For this review, take the finished solid that the model builds, in its own axes (mm). Face numbers are marked on the shaded views. A direction names the side the tool comes from. Coordinates: 2 decimals unless noted, no trailing zeros. Write each loop counter-clockwise with the first axis right and the second up, starting at its lowest first coordinate (ties: lowest second). Pieces come first, ordered by that corner, then holes. Notation, with made-up numbers: M 69,1.5 L 118,1.5 A21 cw 118,25.5 Z; hole C -15.5,61 d4. An arc over 180 degrees is marked long. One line per question, with ' | ' between items.
from build123d import *

# Parameters (mm, degrees)
ESQUISSE2_R             = 65
ESQUISSE2_R_2           = 44
BOSS_EXTRU_1_START      = -47
ESQUISSE3_R             = 112.5
ESQUISSE3_R_2           = 44
BOSS_EXTRU_1_DEPTH      = 47
ENL_V_START             = -10
ESQUISSE4_R             = 112.5
ESQUISSE4_R_2           = 65
ENL_V_MAT_EXTRU_1_DEPTH = 10
ESQUISSE5_R             = 112.5
ESQUISSE5_R_2           = 44
BOSS_EXTRU_2_DEPTH      = 37


with BuildPart() as part:
    # Balayage-Mince1: sweep along a path in Esquisse1
    with BuildLine(Plane(origin=(0, 0, 0), x_dir=(0, 0, -1), z_dir=(1, 0, 0))) as balayage_mince1_path:
        Line((0, 0), (-47, 0))
        ThreePointArc((-47, 0), (-133.103772282, 17.127105185), (-206.099025767, 65.900974233))
        Line((-206.099025767, 65.900974233), (-232.261976671, 92.063925137))
    # Esquisse2 → Balayage-Mince1 (sweep)
    with BuildSketch(Plane.XY):
        Circle(ESQUISSE2_R)
        Circle(ESQUISSE2_R_2, mode=Mode.SUBTRACT)
    sweep(path=balayage_mince1_path.line)

    # Esquisse3 → Boss.-Extru.1 (add)
    with BuildSketch(Plane(origin=(0, 0, 0), x_dir=(-1, 0, 0), z_dir=(0, 0, -1)).offset(BOSS_EXTRU_1_START)):
        Circle(ESQUISSE3_R)
        with Locations(Location((0, 0, 0), (0, 0, 180))):
            Circle(ESQUISSE3_R_2, mode=Mode.SUBTRACT)
    extrude(amount=BOSS_EXTRU_1_DEPTH)

    # Esquisse4 → Enlèv. mat.-Extru.1 (cut)
    with BuildSketch(Plane(origin=(0, 0, 0), x_dir=(-1, 0, 0), z_dir=(0, 0, -1)).offset(ENL_V_START)):
        Circle(ESQUISSE4_R)
        Circle(ESQUISSE4_R_2, mode=Mode.SUBTRACT)
    extrude(amount=ENL_V_MAT_EXTRU_1_DEPTH, mode=Mode.SUBTRACT)

    # Esquisse5 → Boss.-Extru.2 (add)
    with BuildSketch(Plane(origin=(0, 162.162950904, 162.162950904), x_dir=(1, 0, 0), z_dir=(0, 0.7071067811865472, 0.7071067811865478))):
        with Locations(Location((0, -99.134992949, 0), (0, 0, 270))):
            Circle(ESQUISSE5_R)
        with Locations(Location((0, -99.134992949, 0), (0, 0, 270))):
            Circle(ESQUISSE5_R_2, mode=Mode.SUBTRACT)
    extrude(amount=-BOSS_EXTRU_2_DEPTH)


solid = part.part
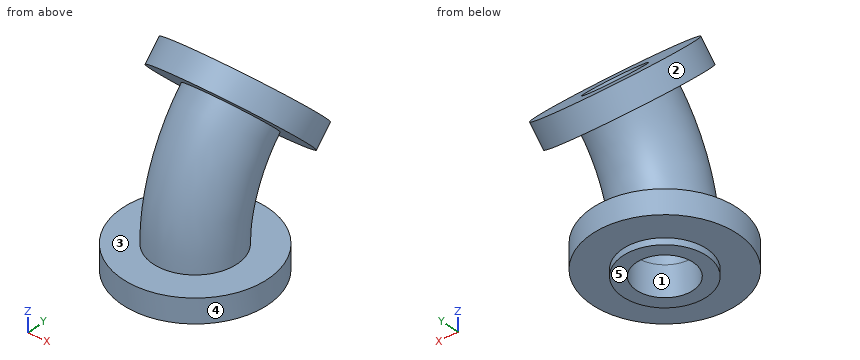
1) We need section A-A on x = 0. State the section outline as (y, z) points, then the cut area to 3 significant figures.
Responses:
outline: M -112.5,10 L -65,10 L -65,0 L -44,0 L -44,47 A269 cw 34.79,237.21 L 60.95,263.37 L 12.51,311.81 L -13.65,285.65 L 19.94,252.06 A290 ccw -65,47 L -112.5,47 Z; M 44,0 L 65,0 L 65,10 L 112.5,10 L 112.5,47 L 65,47 A160 cw 111.86,160.14 L 145.45,126.55 L 171.61,152.71 L 123.18,201.15 L 97.01,174.99 A181 ccw 44,47 Z | area: 18,000 mm^2
2) To check wall thickness, follow line 1 along Y through (x, z) = (0, 19); line 2 along X through (y, z) = (48.5, 169); line 3 along Y through (x, z) = (-15.5, 169.5). State the ranges of each line that lie inside material, in increasing order. Write a range as [from, to].
Responses:
line 1: [-112.5, -44], [44, 112.5] | line 2: [-64.16, -42.74], [42.74, 64.16] | line 3: [-35.79, -11.32], [87.95, 154.83]
3) The part is to be moulded in two halves that separate along X. For the marked faces 1, 2 and 3, say which applies: +X half, -X half, draft (parallel to the pull), parting line (faces both ways), or undercut.
Responses:
face 1: undercut | face 2: parting line | face 3: draft
4) We need section B-B on z = 36. State the section outline as (x, y) points, then the cut area to 3 significant figures.
Responses:
outline: C 0,0 d225; hole C 0,0 d88 | area: 33,700 mm^2
5) Insertion check: pin 1 Ø8 at (x, z) = (12, 117.5) entering from -Y; pin 2 Ø8 at (y, z) = (26.5, 40) entering from -X; pin 3 Ø12 at (x, z) = (48.5, 198.5) entering from -Y. Each pin has a flat end and moves straight along its axis. Give the tip position at first contact, or say it passes through.
Responses:
pin 1: y = -56.35 | pin 2: x = -110.23 | pin 3: y = -4.65
6) We need section D-D on x = -95. State the section outline as (y, z) points, then the cut area to 3 significant figures.
Responses:
outline: M -60.26,10 L 60.26,10 L 60.26,47 L -60.26,47 Z; M 23.29,248.71 L 108.51,163.49 L 134.67,189.65 L 49.45,274.87 Z | area: 8,920 mm^2
7) Machinability: for the marked faces 4 and 5, which of the approach directions +Z, -Z, +X, -X, +Y, -Y give a long, thin tool a straight path to every point of the face, cutting with its end or side? Answer none if there is none.
Responses:
face 4: -Z | face 5: -Z, +X, -X, +Y, -Y
8) We need section C-C on x = 35. State the section outline as (y, z) points, then the cut area to 3 significant figures.
Responses:
outline: M -106.92,10 L -54.77,10 L -54.77,0 L -26.66,0 L -26.66,47 A251.66 cw 47.05,224.95 L 73.21,251.12 L 16.46,307.86 L -9.7,281.7 L 27.17,244.83 A279.77 ccw -54.77,47 L -106.92,47 Z; M 26.66,0 L 54.77,0 L 54.77,10 L 106.92,10 L 106.92,47 L 54.77,47 A170.23 cw 104.63,167.37 L 141.5,130.5 L 167.67,156.66 L 110.92,213.41 L 84.76,187.24 A198.34 ccw 26.66,47 Z | area: 22,400 mm^2
